Build history of the part. All positions in model axes, mm. A direction names the side the tool comes from. Give positions to 0.01 mm unless a question says otherwise; leave off trailing zeros. Loops run counter-clockwise (first coordinate to the right, second up) from the corner with the lowest first, then second, coordinate; pieces in that order, holes last.
1) Band-saw the part on A-A on z = -13.75. List the corners of the cut face in (x, y), then the cut area to 3 significant figures.
2) Band-saw the part on D-D on z = -3.5. List the corners of the cut face in (x, y), then the cut area to 3 significant figures.
3) Band-saw the part on B-B on x = 0. List the corners of the cut face in (y, z), then the cut area to 3 significant figures.
4) 3-axis set-ups, long thin cutter, end or side, ignore diameter. For faces 1 (the cylindrical face through (-0.007, -4.753, -14.732)), 2 (the flat face through (3, -1, -13.5)): which of +Z, -Z, +X, -X, +Y, -Y reach the whole face in a straight line?
5) Flat gauge pins, fed straight in: P1, Ø5, axis at x = -1, z = -11.5, coming from the -Y side; P2, Ø1.5, axis at y = -1.5, z = -6, coming from the +X side; P3, Ø2, axis at x = 2.5, z = -2, coming from the +Y side. Where does each tip first touch, or does it go through?
6) Band-saw the part on C-C on y = -1. List the corners of the cut face in (x, z).
7) Wall check: line 1 (Z direction, x = -4, y = -1.75); line 2 (X direction, y = 3.25, z = -14); line 3 (Y direction, x = 2.75, z = -1). Give the ranges that are in metal, low to high.
Solid Edge part; units mm, degrees
sketch "Sketch1" plane through (0, 0, 0) normal (0, 0, 1) x (1, 0, 0)
  circle A0 centre (0, 0) radius 3
extrude "Protrusion1" add sketch "Sketch1" against normal blind 13.5
sketch "Sketch2" plane through (0, 0, -13.5) normal (0, 0, -1) x (-1, 0, 0)
  line L0 (-3.75, -2.7424) -> (-0.5, -4.6188)
  arc A0 (-0.5, -4.6188) -> (0.5, -4.6188) centre (0, -3.7528) ccw
  line L1 (0.5, -4.6188) -> (3.75, -2.7424)
  arc A1 (3.75, -2.7424) -> (4.25, -1.8764) centre (3.25, -1.8764) ccw
  line L2 (4.25, -1.8764) -> (4.25, 1.8764)
  arc A2 (4.25, 1.8764) -> (3.75, 2.7424) centre (3.25, 1.8764) ccw
  line L3 (3.75, 2.7424) -> (0.5, 4.6188)
  arc A3 (0.5, 4.6188) -> (-0.5, 4.6188) centre (0, 3.7528) ccw
  line L4 (-0.5, 4.6188) -> (-3.75, 2.7424)
  arc A4 (-3.75, 2.7424) -> (-4.25, 1.8764) centre (-3.25, 1.8764) ccw
  line L5 (-4.25, 1.8764) -> (-4.25, -1.8764)
  arc A5 (-3.75, -2.7424) -> (-4.25, -1.8764) centre (-3.25, -1.8764) cw
extrude "ExtrudedProtrusion_2" add sketch "Sketch2" along normal blind 2.5
Findings below:
1. outline: (-4.25, -1.88) arc R1 ccw to (-3.75, -2.74) - (-0.5, -4.62) arc R1 ccw to (0.5, -4.62) - (3.75, -2.74) arc R1 ccw to (4.25, -1.88) - (4.25, 1.88) arc R1 ccw to (3.75, 2.74) - (0.5, 4.62) arc R1 ccw to (-0.5, 4.62) - (-3.75, 2.74) arc R1 ccw to (-4.25, 1.88) - close
1. area: 62.2 mm2
2. outline: circle Ø6 at (0, 0)
2. area: 28.3 mm2
3. outline: (-4.75, -16) - (4.75, -16) - (4.75, -13.5) - (3, -13.5) - (3, 0) - (-3, 0) - (-3, -13.5) - (-4.75, -13.5) - close
3. area: 105 mm2
4. face 1: +Z, -Z, -Y
4. face 2: +Z
5. P1: stops at y = -4.75
5. P2: stops at x = 2.9
5. P3: stops at y = 2.6
6. outline: (-4.25, -16) - (4.25, -16) - (4.25, -13.5) - (2.83, -13.5) - (2.83, 0) - (-2.83, 0) - (-2.83, -13.5) - (-4.25, -13.5) - close
7. line 1: z = -16 to -13.5
7. line 2: x = -2.87 to 2.87
7. line 3: y = -1.2 to 1.2
